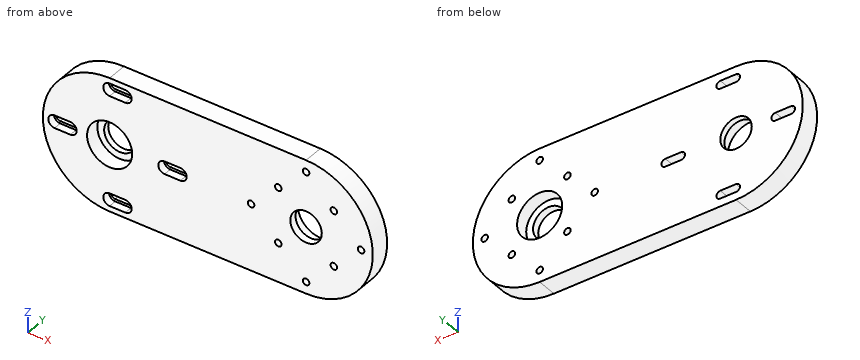
from build123d import *

# Parameters (mm, degrees)
SKETCH1_R           = 10
SKETCH1_R_2         = 2.1
BOSS_EXTRUDE1_DEPTH = 12.7
SKETCH2_R           = 14.35
CUT_EXTRUDE1_DEPTH  = 8.1
CUT_EXTRUDE2_START  = -12.7
SKETCH3_R           = 14.35
CUT_EXTRUDE2_DEPTH  = 9.1
CUT_EXTRUDE3_START  = -12.7
CUT_EXTRUDE3_DEPTH  = 5


with BuildPart() as part:
    # Sketch1 → Boss-Extrude1 (new body)
    with BuildSketch(Plane(origin=(0, 0, 0), x_dir=(1, 0, 0), z_dir=(0, 1, 0))):
        with BuildLine():
            ThreePointArc((-125, 42.5), (-167.5, 0), (-125, -42.5))
            Line((-125, -42.5), (0, -42.5))
            ThreePointArc((0, -42.5), (42.5, 0), (0, 42.5))
            Line((0, 42.5), (-125, 42.5))
        make_face()
        with BuildLine():
            Line((-90, 2.5), (-80, 2.5))
            ThreePointArc((-80, 2.5), (-77.5, 0), (-80, -2.5))
            Line((-80, -2.5), (-90, -2.5))
            ThreePointArc((-90, -2.5), (-92.5, 0), (-90, 2.5))
        make_face(mode=Mode.SUBTRACT)
        with BuildLine():
            ThreePointArc((-125, -37.5), (-127.5, -35), (-125, -32.5))
            Line((-125, -32.5), (-115, -32.5))
            ThreePointArc((-115, -32.5), (-112.5, -35), (-115, -37.5))
            Line((-115, -37.5), (-125, -37.5))
        make_face(mode=Mode.SUBTRACT)
        with BuildLine():
            ThreePointArc((-160, -2.5), (-162.5, 0), (-160, 2.5))
            Line((-160, 2.5), (-150, 2.5))
            ThreePointArc((-150, 2.5), (-147.5, 0), (-150, -2.5))
            Line((-150, -2.5), (-160, -2.5))
        make_face(mode=Mode.SUBTRACT)
        with Locations(Location((-125, 0, 0), (0, 0, 270))):
            Circle(SKETCH1_R, mode=Mode.SUBTRACT)
        with BuildLine():
            ThreePointArc((-125, 32.5), (-127.5, 35), (-125, 37.5))
            Line((-125, 37.5), (-115, 37.5))
            ThreePointArc((-115, 37.5), (-112.5, 35), (-115, 32.5))
            Line((-115, 32.5), (-125, 32.5))
        make_face(mode=Mode.SUBTRACT)
        with Locations(Location((0, 35, 0), (0, 0, 270))):
            Circle(SKETCH1_R_2, mode=Mode.SUBTRACT)
        with Locations(Location((0, -35, 0), (0, 0, 270))):
            Circle(SKETCH1_R_2, mode=Mode.SUBTRACT)
        with Locations(Location((-17.67766953, -17.67766953, 0), (0, 0, 270))):
            Circle(SKETCH1_R_2, mode=Mode.SUBTRACT)
        with Locations(Location((17.67766953, -17.67766953, 0), (0, 0, 270))):
            Circle(SKETCH1_R_2, mode=Mode.SUBTRACT)
        with Locations(Location((-35, 0, 0), (0, 0, 270))):
            Circle(SKETCH1_R_2, mode=Mode.SUBTRACT)
        with Locations(Location((-17.67766953, 17.67766953, 0), (0, 0, 270))):
            Circle(SKETCH1_R_2, mode=Mode.SUBTRACT)
        with Locations(Location((0, 0, 0), (0, 0, 270))):
            Circle(SKETCH1_R, mode=Mode.SUBTRACT)
        with Locations(Location((35, 0, 0), (0, 0, 270))):
            Circle(SKETCH1_R_2, mode=Mode.SUBTRACT)
        with Locations(Location((17.67766953, 17.67766953, 0), (0, 0, 270))):
            Circle(SKETCH1_R_2, mode=Mode.SUBTRACT)
    extrude(amount=-BOSS_EXTRUDE1_DEPTH)

    # Sketch2 → Cut-Extrude1 (cut)
    with BuildSketch(Plane(origin=(0, 0, 0), x_dir=(1, 0, 0), z_dir=(0, 1, 0))):
        with Locations(Location((0, 0, 0), (0, 0, 270))):
            Circle(SKETCH2_R)
    extrude(amount=-CUT_EXTRUDE1_DEPTH, mode=Mode.SUBTRACT)

    # Sketch3 → Cut-Extrude2 (cut)
    with BuildSketch(Plane(origin=(0, 0, 0), x_dir=(1, 0, 0), z_dir=(0, 1, 0)).offset(CUT_EXTRUDE2_START)):
        with Locations(Location((-125, 0, 0), (0, 0, 270))):
            Circle(SKETCH3_R)
    extrude(amount=CUT_EXTRUDE2_DEPTH, mode=Mode.SUBTRACT)

    # Sketch4 → Cut-Extrude3 (cut)
    with BuildSketch(Plane(origin=(0, 0, 0), x_dir=(1, 0, 0), z_dir=(0, 1, 0)).offset(CUT_EXTRUDE3_START)):
        with BuildLine():
            Line((-150, -4.05), (-160, -4.05))
            ThreePointArc((-160, -4.05), (-164.05, 0), (-160, 4.05))
            Line((-160, 4.05), (-150, 4.05))
            ThreePointArc((-150, 4.05), (-145.95, 0), (-150, -4.05))
        make_face()
        with BuildLine():
            Line((-125, -30.95), (-115, -30.95))
            ThreePointArc((-115, -30.95), (-110.95, -35), (-115, -39.05))
            Line((-115, -39.05), (-125, -39.05))
            ThreePointArc((-125, -39.05), (-129.05, -35), (-125, -30.95))
        make_face()
        with BuildLine():
            Line((-80, -4.05), (-90, -4.05))
            ThreePointArc((-90, -4.05), (-94.05, 0), (-90, 4.05))
            Line((-90, 4.05), (-80, 4.05))
            ThreePointArc((-80, 4.05), (-75.95, 0), (-80, -4.05))
        make_face()
        with BuildLine():
            Line((-125, 39.05), (-115, 39.05))
            ThreePointArc((-115, 39.05), (-110.95, 35), (-115, 30.95))
            Line((-115, 30.95), (-125, 30.95))
            ThreePointArc((-125, 30.95), (-129.05, 35), (-125, 39.05))
        make_face()
    extrude(amount=CUT_EXTRUDE3_DEPTH, mode=Mode.SUBTRACT)


solid = part.part
Verification items for the finished model (mm, model axes). Coordinates: 2 decimals unless noted, no trailing zeros. Order: outer loops, then holes, each group sorted by start corner. A loop starts at its lowest first (then second) coordinate and runs counter-clockwise, first axis right, second up. Notation, with made-up numbers: (-27.75, 41.25) -> (10.25, 41.25) arc R24 cw to (10.25, 52.25) -> close; hole circle Ø2 at (-2, 35). An arc over 180 degrees is marked (long way). Put each result on its own line as item: value. Start each with the question number.
1. Cross-section at A-A, the plane x = -35. Record the boundary of the cut face in (y, z), then the cut area to 3 significant figures.
2. Material ranges on L1, parallel to X at y = -0.75, z = -6; L2, parallel to X at y = -8.5, z = 19; L3, parallel to Z at x = -8, y = -1.75, recorded low to high. Write a range as [from, to].
3. Go/stop test with flat-tipped pins: pin 1 Ø2 at (x, y) = (20, -4) entering from +Z; pin 2 Ø6 at (y, z) = (-9.5, 14.5) entering from +X; pin 3 Ø4 at (x, z) = (-35, 0) entering from +Y; pin 4 Ø2.5 at (x, y) = (-153.5, -9.5) entering from +Z. Record where each tip stops, or that it passes through.
4. Cross-section at B-B, the plane y = -10.5. Count the separate pieces of the cut face and the enclosed holes in it, then the cut area to 3 significant figures.
Computed:
1. outline: (-12.7, -42.5) -> (0, -42.5) -> (0, -2.1) -> (-12.7, -2.1) -> close; (-12.7, 2.1) -> (0, 2.1) -> (0, 42.5) -> (-12.7, 42.5) -> close
1. area: 1,030 mm2
2. L1: [-167.07, -133], [-117, -13.04], [13.04, 42.07]
2. L2: [-163.02, -19.31], [-16.05, 16.05], [19.31, 38.02]
2. L3: [-42.5, -11.91], [11.91, 42.5]
3. pin 1: z = 38.02
3. pin 2: x = 40.91
3. pin 3: through
3. pin 4: z = 32.61
4. separate pieces: 1
4. enclosed holes: 14
4. area: 14,700 mm2
